Geometry: see drawing. Coordinates: mm, zero at the bounding-box minimum. Give positions to 0.01 mm unless a question says otherwise; leave off trailing zeros. Write each loop counter-clockwise with the first axis right and the second up, starting at its lowest first coordinate (ties: lowest second). Pieces come first, ordered by that corner, then holes. Notation, with made-up numbers: (77.25, 6) - (102.25, 6) arc R14 ccw to (102.25, 14) - close; hole circle Ø4 at (53, -36.75). An arc over 180 degrees is marked (long way). Return JSON: item names as keys, results as strings.
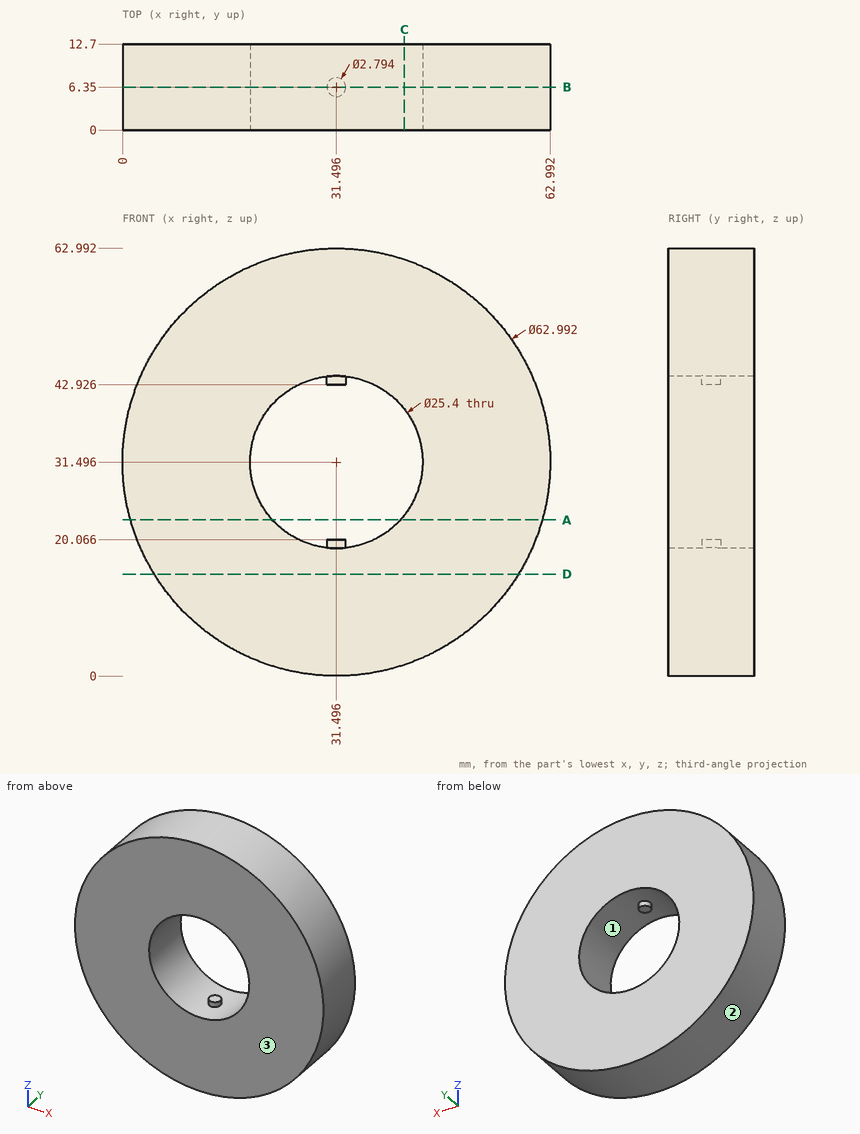
Q1. Pin query (flat end, axial travel): P1, Ø2, axis at x = 40.5, y = 9.5, coming from the -Z side; P2, Ø1.5, axis at x = 45, y = 3, coming from the +Z side; P3, Ø2, axis at y = 5.5, z = 22.5, coming from the -X side. Return the tip coordinate at first contact, or that it passes through.
Answer key:
{"P1": "stops at z = 1.03", "P2": "stops at z = 60.29", "P3": "stops at x = 1.03"}
Q2. Section query B-B, the plane y = 6.35. Return the cut outline in (x, z), plus the area to 3 significant figures.
Answer key:
{"outline": "circle Ø62.99 at (31.5, 31.5); hole (30.1, 18.87) - (30.1, 20.07) - (32.89, 20.07) - (32.89, 18.87) arc R12.7 ccw to (32.89, 44.12) - (32.89, 42.93) - (30.1, 42.93) - (30.1, 44.12) arc R12.7 ccw to start", "area": "2,620 mm^2"}
Q3. Section query C-C, the plane x = 41.5. Return the cut outline in (y, z).
Answer key:
{"outline": "(0, 1.63) - (12.7, 1.63) - (12.7, 23.67) - (0, 23.67) - close; (0, 39.32) - (12.7, 39.32) - (12.7, 61.36) - (0, 61.36) - close"}
Q4. Mould query, pull axis X, two halves, no side actions, for the marked faces 1, 2 and 3. Classes: pulls with the +X half, pulls with the -X half, needs draft (parallel to the pull), parting line crosses it, or undercut.
Answer key:
{"face 1": "undercut", "face 2": "parting line crosses it", "face 3": "needs draft"}
Q5. Section query A-A, the plane z = 23. Return the cut outline in (x, y), plus the area to 3 significant figures.
Answer key:
{"outline": "(1.17, 0) - (22.06, 0) - (22.06, 12.7) - (1.17, 12.7) - close; (40.94, 0) - (61.82, 0) - (61.82, 12.7) - (40.94, 12.7) - close", "area": "531 mm^2"}
Q6. Material intervals for probe 1 along X at (y, z) = (11.25, 32); probe 2 along Z at (x, y) = (32, 6.25); probe 3 along X at (y, z) = (5.25, 35), sorted ascending. Write a range as [from, to].
Answer key:
{"probe 1": "x = [0, 18.81], [44.19, 62.99]", "probe 2": "z = [0, 20.07], [42.93, 62.99]", "probe 3": "x = [0.2, 19.29], [43.7, 62.8]"}
Q7. Section query D-D, the plane z = 15. Return the cut outline in (x, y), plus the area to 3 significant figures.
Answer key:
{"outline": "(4.67, 0) - (58.33, 0) - (58.33, 12.7) - (4.67, 12.7) - close", "area": "681 mm^2"}
